The model under review builds one solid part; all positions refer to its coordinate system, in mm. Round coordinates to 2 decimals unless told otherwise and drop trailing zeros. Write each loop counter-clockwise with the first axis right and the second up, starting at its lowest first coordinate (ties: lowest second). Pieces come first, ordered by that corner, then holes. Notation, with made-up numbers: (-16.5, -25.5) - (38.5, -25.5) arc R16 ccw to (38.5, -7.5) - close; hole circle Ø5 at (74, -34.75). An arc over 180 degrees is marked (long way). Return JSON: item names as keys, results as strings.
from build123d import *

# Parameters (mm, degrees)
SKETCH1_R           = 2.5
BOSS_EXTRUDE1_DEPTH = 200
FILLET1_R           = 1.065
FILLET2_R           = 2.13


with BuildPart() as part:
    # Sketch1 → Boss-Extrude1 (new body)
    with BuildSketch(Plane.YZ):
        Polygon((-12.5, -3.25), (-12.5, -12.5), (-3.25, -12.5), (-3.25, -10.37), (-8.863862556, -10.37), (-2.873862556, -4.38), (2.873862556, -4.38), (8.863862556, -10.37), (3.25, -10.37), (3.25, -12.5), (12.5, -12.5), (12.5, -3.25), (10.37, -3.25), (10.37, -8.863862556), (4.38, -2.873862556), (4.38, 2.873862556), (10.37, 8.863862556), (10.37, 3.25), (12.5, 3.25), (12.5, 12.5), (3.25, 12.5), (3.25, 10.37), (8.863862556, 10.37), (2.873862556, 4.38), (-2.873862556, 4.38), (-8.863862556, 10.37), (-3.25, 10.37), (-3.25, 12.5), (-12.5, 12.5), (-12.5, 3.25), (-10.37, 3.25), (-10.37, 8.863862556), (-4.38, 2.873862556), (-4.38, -2.873862556), (-10.37, -8.863862556), (-10.37, -3.25), align=None)
        with Locations(Location((0, 0, 0), (0, 0, 270))):
            Circle(SKETCH1_R, mode=Mode.SUBTRACT)
    extrude(amount=BOSS_EXTRUDE1_DEPTH)

    # Fillet1
    fillet1_edges = [part.edges().sort_by_distance(p)[0] for p in [
        (100, -10.37, -8.863862556),
        (100, 2.873862556, -4.38),
        (100, -2.873862556, -4.38),
        (100, -4.38, 2.873862556),
        (100, -4.38, -2.873862556),
        (100, -2.873862556, 4.38),
        (100, 2.873862556, 4.38),
        (100, 4.38, 2.873862556),
        (100, 4.38, -2.873862556),
        (100, -8.863862556, -10.37),
        (100, 8.863862556, -10.37),
        (100, 10.37, -8.863862556),
        (100, -10.37, 8.863862556),
        (100, -8.863862556, 10.37),
        (100, 10.37, 8.863862556),
        (100, 8.863862556, 10.37),
        (100, 12.5, 3.25),
        (100, -3.25, -12.5),
        (100, -10.37, 3.25),
        (100, 10.37, 3.25),
        (100, -10.37, -3.25),
        (100, -12.5, -3.25),
        (100, -12.5, 3.25),
        (100, 3.25, -10.37),
        (100, -3.25, -10.37),
        (100, 3.25, -12.5),
        (100, 10.37, -3.25),
        (100, 12.5, -3.25),
        (100, 3.25, 12.5),
        (100, 3.25, 10.37),
        (100, -3.25, 10.37),
        (100, -3.25, 12.5),
    ]]
    fillet(fillet1_edges, radius=FILLET1_R - 0.0001)  # a hair under: the kernel refuses the full size

    # Fillet2
    fillet2_edges = [part.edges().sort_by_distance(p)[0] for p in [
        (100, -12.5, 12.5),
        (100, 12.5, 12.5),
        (100, 12.5, -12.5),
        (100, -12.5, -12.5),
    ]]
    fillet(fillet2_edges, radius=FILLET2_R)


solid = part.part
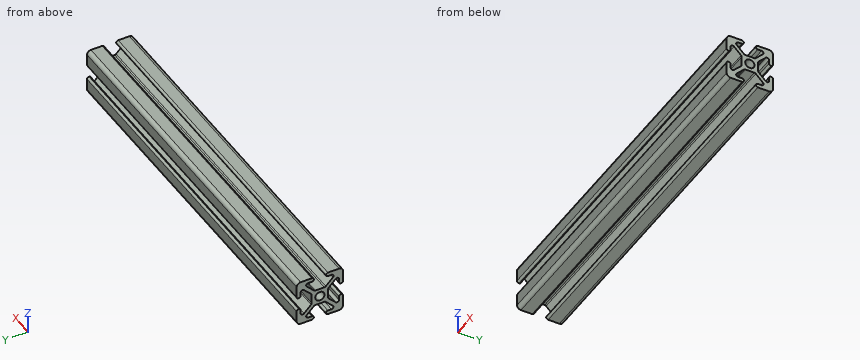
(1) Clearance check with flat-ended pins moving along their axes: pin 1 Ø3 at (x, y) = (74.5, -1.5) entering from +Z; pin 2 Ø4 at (x, z) = (60.5, 0) entering from -Y; pin 3 Ø2.5 at (x, y) = (89, 0) entering from -Z. State where each tip first meets the part, or that it passes through.
Filled in:
{"pin 1": "stops at z = 4.54", "pin 2": "stops at y = -4.38", "pin 3": "stops at z = -4.38"}
(2) Add section A-A (y = 0). Write out the cut boundary in (x, z), plus the area to 3 significant figures.
Filled in:
{"outline": "(0, -4.38) - (200, -4.38) - (200, -2.5) - (0, -2.5) - close; (0, 2.5) - (200, 2.5) - (200, 4.38) - (0, 4.38) - close", "area": "752 mm2"}
(3) Wall thickness on line 1 (Z direction, x = 77, y = 4); line 2 (Y direction, x = 158, z = -6.25); line 3 (Z direction, x = 185.5, y = 9.5): over which ranges is each line inside the solid? List them lowest first.
Filled in:
{"line 1": "z = -12.45 to -10.42, -5.51 to 5.51, 10.42 to 12.45", "line 2": "y = -12.5 to -10.37, -7.76 to -4.74, 4.74 to 7.76, 10.37 to 12.5", "line 3": "z = -12.5 to -7.34, 7.34 to 12.5"}
